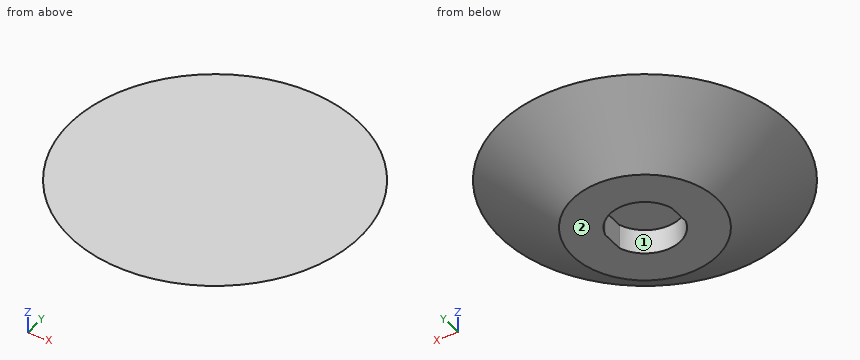
```python
from build123d import *

# Parameters (mm, degrees)
CUT_EXTRUDE_1_DEPTH = 34.3


with BuildPart() as part:
    # 草图3 → 旋转1 (revolve)
    with BuildSketch(Plane(origin=(0, 0, 0), x_dir=(1, 0, 0), z_dir=(0, 1, 0))):
        Polygon((-100, 36.733070518), (0, 36.733070518), (0, -33.266929482), (-200, -33.266929482), align=None)
    revolve(axis=Axis((0, 0, -36.733070518), (0, 0, 1)))

    # 草图4 → 切除-拉伸1 (cut)
    with BuildSketch(Plane(origin=(0, 0, -36.733070518), x_dir=(-1, 0, 0), z_dir=(0, 0, -1))):
        with BuildLine():
            Line((-46.25, 13.747727085), (-46.25, -16.046690113))
            ThreePointArc((-46.25, -16.046690113), (0, -48.954660285), (46.25, -16.046690113))
            Line((46.25, -16.046690113), (46.25, 13.747727085))
            ThreePointArc((46.25, 13.747727085), (0, 48.25), (-46.25, 13.747727085))
        make_face()
    extrude(amount=-CUT_EXTRUDE_1_DEPTH, mode=Mode.SUBTRACT)


solid = part.part
```
Could you check a few things on this model? Use its own coordinates, in mm. Face numbers are marked on the shaded views. A direction names the side the tool comes from. Round coordinates to 2 decimals unless told otherwise and drop trailing zeros. Loops run counter-clockwise (first coordinate to the right, second up) from the corner with the lowest first, then second, coordinate; pieces in that order, holes last. Notation, with made-up numbers: (30.25, 83.5) - (38.25, 83.5) arc R18 cw to (38.25, 108.5) - close; hole circle Ø8 at (-22.75, 33.25). An arc over 180 degrees is marked (long way). Answer in a Markdown table with one row per item. Add a question column.
(1) I need wall thicknesses on line 1 along X through (y, z) = (-26, -28); line 2 along X through (y, z) = (-2.5, -25); line 3 along Y through (x, z) = (-27.5, -5). Which ranges of each line are inside material? Lowest first, please.
(2) If we section it at C-C (z = 16): Please give me the cut outline in (x, y).
(3) I'm going to push flat-ended pins straight in: pin 1 (3 mm diameter, centred on y = 5.5, z = 19, fed in from -X); pin 2 (6 mm diameter, centred on y = -74.5, z = 18.5, fed in from -X); pin 3 (4 mm diameter, centred on y = 57, z = -26.5, fed in from -X). Where does each tip first touch, or does it pass through?
(4) If we section it at B-B (y = 0): Please give me the cut outline in (x, z).
(5) For the marked faces 1 and 2, which set-ups out of +Z, -Z, +X, -X, +Y, -Y let a thin tool reach every point of the face, with its end or its side?
(6) If we section it at A-A (x = 0): Please give me the cut outline in (y, z), plus the area to 3 significant figures.
Model answer:
| question | item | result |
|---|---|---|
| 1 | line 1 | x = -109.43 to -41.48, 41.48 to 109.43 |
| 1 | line 2 | x = -116.73 to -46.25, 46.25 to 116.73 |
| 1 | line 3 | y = -142.71 to -40.5, 39.65 to 142.71 |
| 2 | outline | circle Ø350.67 at (0, 0) |
| 3 | pin 1 | stops at x = -181.68 |
| 3 | pin 2 | stops at x = -167.54 |
| 3 | pin 3 | stops at x = -102.9 |
| 4 | outline | (-200, 33.27) - (-100, -36.73) - (-46.25, -36.73) - (-46.25, -2.43) - (46.25, -2.43) - (46.25, -36.73) - (100, -36.73) - (200, 33.27) - close |
| 5 | face 1 | -Z |
| 5 | face 2 | -Z, +X, -X, +Y, -Y |
| 6 | outline | (-200, 33.27) - (-100, -36.73) - (-48.95, -36.73) - (-48.95, -2.43) - (48.25, -2.43) - (48.25, -36.73) - (100, -36.73) - (200, 33.27) - close |
| 6 | area | 17,700 mm² |
